```python
from build123d import *

# Parameters (mm, degrees)
F0_R     = 6
F1_DEPTH = 1
F3_DEPTH = 4


with BuildPart() as f1:
    # F0 (on Top) → F1 (new body)
    with BuildSketch(Plane.XY):
        Circle(F0_R)
    extrude(amount=F1_DEPTH)

    # F2 (on Front) → F3 (join, symmetric)
    with BuildSketch(Plane.XZ):
        Polygon((0.65, 4), (0.65, 1), (2, 1), (0.65, 5), align=None)
        Polygon((-0.65, 5), (-2, 1), (-0.65, 1), (-0.65, 4), align=None)
        with BuildLine():
            ThreePointArc((-0.65, 4), (-0.645, 4.5), (-0.65, 5))
            Line((-0.65, 5), (-0.65, 4))
        make_face()
        with BuildLine():
            ThreePointArc((0.65, 5), (0.645, 4.5), (0.65, 4))
            Line((0.65, 4), (0.65, 5))
        make_face()
    extrude(amount=F3_DEPTH, both=True)


solid = f1.part
```
Geometry: final body of the model. Coordinates: model frame, mm. A direction names the side the tool comes from. Give positions to 0.01 mm unless a question says otherwise; leave off trailing zeros. Loops run counter-clockwise (first coordinate to the right, second up) from the corner with the lowest first, then second, coordinate; pieces in that order, holes last. Notation, with made-up numbers: (7, 56) -> (30, 56) arc R10 ccw to (30, 66) -> close; hole circle Ø1 at (1.5, 40). An arc over 180 degrees is marked (long way). Return JSON: item names as keys, results as strings.
Item 1: Pin query (flat end, axial travel): P1, Ø2.5, axis at y = 0.5, z = 3, coming from the +X side; P2, Ø1.1, axis at x = 1.5, z = 3, coming from the +Y side; P3, Ø1, axis at y = 3.5, z = 3, coming from the -X side; P4, Ø1.5, axis at x = -4.5, z = 3, coming from the -Y side. Return the tip coordinate at first contact, or that it passes through.
Filled in:
{"P1": "x = 1.75", "P2": "y = 4", "P3": "x = -1.49", "P4": "through"}
Item 2: Mould query, pull axis X, two halves, no side actions, for faces 5 (the cylindrical face through (-5.994, 0.264, 0.493)), 6 (the flat face through (-1, -4, 2)), 7 (the cylindrical face through (-0.645, -0.056, 4.493)), 8 (the flat face through (1.334, 0.056, 2.972)). Classes: released by +X, released by -X, zero draft, split by the parting line, or undercut.
Filled in:
{"face 5": "split by the parting line", "face 6": "zero draft", "face 7": "undercut", "face 8": "released by +X"}
Item 3: Section D-D, the plane z = 3.5. Output: boundary loops of the cut face in (x, y), plus the area to 3 significant figures.
Filled in:
{"outline": "(-1.16, -4) -> (-0.65, -4) -> (-0.65, 4) -> (-1.16, 4) -> close; (0.65, -4) -> (1.16, -4) -> (1.16, 4) -> (0.65, 4) -> close", "area": "8.10 mm^2"}
Item 4: Section C-C, the plane x = 1.75. Output: boundary loops of the cut face in (y, z).
Filled in:
{"outline": "(-5.74, 0) -> (5.74, 0) -> (5.74, 1) -> (4, 1) -> (4, 1.74) -> (-4, 1.74) -> (-4, 1) -> (-5.74, 1) -> close"}
Item 5: Line query: line 1 (Z direction, x = 0.5, y = 2); line 2 (Y direction, x = -1.25, z = 1.6); line 3 (X direction, y = 0.25, z = 4.5) (3 decimals). Output: solid intervals per line, ascending.
Filled in:
{"line 1": "0 to 1", "line 2": "-4 to 4", "line 3": "-0.819 to -0.645, 0.645 to 0.819"}
Item 6: Section B-B, the plane z = 1.3. Output: boundary loops of the cut face in (x, y), plus the area to 3 significant figures.
Filled in:
{"outline": "(-1.9, -4) -> (-0.65, -4) -> (-0.65, 4) -> (-1.9, 4) -> close; (0.65, -4) -> (1.9, -4) -> (1.9, 4) -> (0.65, 4) -> close", "area": "20.0 mm^2"}
Item 7: Access query for faces 1 (the flat face through (-1, 4, 2)), 2 (the flat face through (1, -4, 3)), 3 (the flat face through (0, 0, 0)), 4 (the flat face through (-1.316, -0.056, 3.028)). Directions: +Z, -Z, +X, -X, +Y, -Y. A direction counts if a zero-diameter tool reaches every point of the face in a straight line with its end or side. Return the directions, or none.
Filled in:
{"face 1": "+Z, +X, -X, +Y", "face 2": "+Z, +X, -X, -Y", "face 3": "-Z, +X, -X, +Y, -Y", "face 4": "+Z, -X, +Y, -Y"}
